Autodesk Fusion 360 part; units mm, degrees
sketch "lcd" plane through (0, 0, 0) normal (0, 1, 0) x (1, 0, 0)
  line L0 (53, -34) -> (-53, -34)
  line L1 (-53, -34) -> (-53, 34)
  line L2 (-53, 34) -> (53, 34)
  line L3 (53, 34) -> (53, -34)
  line L4 (53, -34) -> (-53, 34) construction
  line L5 (-53, -34) -> (53, 34) construction
  line L6 (49.65, -30.9) -> (-49.65, -30.9) construction
  line L7 (-49.65, -30.9) -> (-49.65, 30.9) construction
  line L8 (-49.65, 30.9) -> (49.65, 30.9) construction
  line L9 (49.65, 30.9) -> (49.65, -30.9) construction
  line L10 (49.65, -30.9) -> (-49.65, 30.9) construction
  line L11 (-49.65, -30.9) -> (49.65, 30.9) construction
  circle A0 centre (-49.65, 30.9) radius 1.5
  circle A1 centre (-49.65, 30.9) radius 2.5
  circle A2 centre (-49.65, -30.9) radius 2.5
  circle A3 centre (-49.65, -30.9) radius 1.5
  circle A4 centre (49.65, -30.9) radius 2.5
  circle A5 centre (49.65, -30.9) radius 1.5
  circle A6 centre (49.65, 30.9) radius 2.5
  circle A7 centre (49.65, 30.9) radius 1.5
  circle A8 centre (-27.38, -24.54) radius 2.5
  circle A9 centre (-27.38, -24.54) radius 1.5
  circle A10 centre (30.62, -24.54) radius 1.5
  circle A11 centre (30.62, -24.54) radius 2.5
  circle A12 centre (-27.38, 24.5) radius 1.5
  circle A13 centre (-27.38, 24.5) radius 2.5
  circle A14 centre (30.62, 24.5) radius 2.5
  circle A15 centre (30.62, 24.5) radius 1.5
  line L12 (48.5612, 7.0715) -> (50.7124, 7.0715)
  line L13 (50.7124, 7.0715) -> (50.7124, -8.2737)
  line L14 (50.7124, -8.2737) -> (48.5612, -8.2737)
  line L15 (48.5612, -8.2737) -> (48.5612, 7.0715)
  dimension "d1" = 106
  dimension "d2" = 68
  dimension "d3" = 99.3
  dimension "d4" = 61.8
  dimension "d5" = 3
  dimension "d6" = 5
  dimension "d7" = 3
  dimension "d8" = 5
  dimension "d9" = 3
  dimension "d10" = 5
  dimension "d11" = 3
  dimension "d12" = 5
  dimension "d13" = 3
  dimension "d14" = 5
  dimension "d15" = 9.46
  dimension "d16" = 25.62
  dimension "d17" = 3
  dimension "d18" = 5
  dimension "d19" = 22.38
  dimension "d20" = 3
  dimension "d21" = 5
  dimension "d22" = 3
  dimension "d23" = 5
  dimension "d24" = 9.5
  dimension "d25" = 9.5
extrude "Extrude1" add sketch "lcd" against normal blind 8.6 contours L0 L1 L2 L3 | A0 | A1 | A2 | A3 | A4 | A5 | A6 | A7 | A8 | A9 | A10 | A11 | A12 | A13 | A14 | A15 | L12 L13 L14 L15
extrude "Extrude2" add sketch "lcd" along normal blind 4 contours A1 | A2 | A4 | A6 | A8 | A11 | A13 | A14
extrude "Extrude3" add sketch "lcd" along normal blind 5 contours L12 L13 L14 L15
The model under review builds one solid part; all positions refer to its coordinate system, in mm. A direction names the side the tool comes from. Give positions to 0.01 mm unless a question says otherwise; leave off trailing zeros. Loops run counter-clockwise (first coordinate to the right, second up) from the corner with the lowest first, then second, coordinate; pieces in that order, holes last. Notation, with made-up numbers: (17, -36) -> (29, -36) arc R18 ccw to (29, -9) -> close; hole circle Ø1 at (-18.75, 2). An arc over 180 degrees is marked (long way). Answer as a JSON object with one key per item and string values. Group by question number.
Q1. Take a section at B-B (z = -4). Write out the cut boundary in (x, y).
Q2. Take a section at D-D (z = -24.5). Write out the cut boundary in (x, y), plus the area to 3 significant figures.
Q3. Take a section at C-C (x = 49.65). Write out the cut boundary in (y, z), plus the area to 3 significant figures.
Q4. Tool access review of faces 5 (the flat face through (50, 2, -7.072)), 6 (the flat face through (50, 4, -29)), 7 (the flat face through (31, 0, -25)): name each direction out of +Z, -Z, +X, -X, +Y, -Y from which nothing blocks a thin tool from reaching the whole face with its end or side.
Q5. Take a section at A-A (x = -49.65). Write out the cut boundary in (y, z), plus the area to 3 significant figures.
Q6. Wall thickness on line 1 along X through (y, z) = (1.75, 30.9); line 2 along X through (y, z) = (2.45, 24.54); line 3 along Z through (x, y) = (-27.38, 1.2): over which ranges is each line inside the solid? List them lowest first.
Q7. Insertion check: pin 1 (8 mm diameter, centred on y = 0.5, z = 11.5, fed in from +X); pin 2 (2.5 mm diameter, centred on x = 31.5, z = -25.5, fed in from +Y); pin 3 (1.5 mm diameter, centred on x = 50, z = -31.5, fed in from +Y); pin 4 (1.1 mm diameter, centred on x = 49.5, y = 2.5, fed in from -Z). Each pin has a flat end and moves straight along its axis. Give the tip position at first contact, or say it passes through.
Q8. Draft analysis for pull direction X (two halves, no side actions). For faces 1 (the cylindrical face through (51.036, 1.972, -31.475)), 2 (the flat face through (50.712, 2, 0)), 3 (the flat face through (50, 0, 31)), 4 (the flat face through (-26, 4, -23)), state which applies: pulls with the +X half, pulls with the -X half, needs draft (parallel to the pull), parting line crosses it, or undercut.
Answer below:
{
 "1": {"outline": "(-53, -8.6) -> (53, -8.6) -> (53, 0) -> (50.71, 0) -> (50.71, 5) -> (48.56, 5) -> (48.56, 0) -> (-53, 0) -> close"},
 "2": {"outline": "(-53, -8.6) -> (53, -8.6) -> (53, 0) -> (33.12, 0) -> (33.12, 4) -> (32.12, 4) -> (32.12, 0) -> (29.12, 0) -> (29.12, 4) -> (28.12, 4) -> (28.12, 0) -> (-24.88, 0) -> (-24.88, 4) -> (-25.88, 4) -> (-25.88, 0) -> (-28.88, 0) -> (-28.88, 4) -> (-29.88, 4) -> (-29.88, 0) -> (-53, 0) -> close", "area": "928 mm2"},
 "3": {"outline": "(-8.6, -34) -> (0, -34) -> (0, -33.4) -> (4, -33.4) -> (4, -32.4) -> (0, -32.4) -> (0, -29.4) -> (4, -29.4) -> (4, -28.4) -> (0, -28.4) -> (0, -7.07) -> (5, -7.07) -> (5, 8.27) -> (0, 8.27) -> (0, 28.4) -> (4, 28.4) -> (4, 29.4) -> (0, 29.4) -> (0, 32.4) -> (4, 32.4) -> (4, 33.4) -> (0, 33.4) -> (0, 34) -> (-8.6, 34) -> close", "area": "678 mm2"},
 "4": {"face 5": "+X, -X, +Y", "face 6": "-Z, +X, -X, +Y", "face 7": "+Y"},
 "5": {"outline": "(-8.6, -34) -> (0, -34) -> (0, -33.4) -> (4, -33.4) -> (4, -32.4) -> (0, -32.4) -> (0, -29.4) -> (4, -29.4) -> (4, -28.4) -> (0, -28.4) -> (0, 28.4) -> (4, 28.4) -> (4, 29.4) -> (0, 29.4) -> (0, 32.4) -> (4, 32.4) -> (4, 33.4) -> (0, 33.4) -> (0, 34) -> (-8.6, 34) -> close", "area": "601 mm2"},
 "6": {"line 1": "x = -52.15 to -51.15, -48.15 to -47.15, 47.15 to 48.15, 51.15 to 52.15", "line 2": "x = -29.88 to -28.88, -25.88 to -24.88, 28.12 to 29.12, 32.12 to 33.12", "line 3": "z = -27 to -26, -23 to -22, 22.04 to 23.04, 26.04 to 27.04"},
 "7": {"pin 1": "stops at x = 53", "pin 2": "stops at y = 4", "pin 3": "stops at y = 0", "pin 4": "stops at z = -33.4"},
 "8": {"face 1": "undercut", "face 2": "pulls with the +X half", "face 3": "undercut", "face 4": "needs draft"}
}
